from build123d import *

# Parameters (mm, degrees)
BOSS_EXTRUDE1_DEPTH = 6.25
SKETCH2_R           = 10
SKETCH2_R_2         = 5
BOSS_EXTRUDE2_DEPTH = 3
BOSS_EXTRUDE2_DRAFT = 10
SKETCH3_R           = 5
SKETCH3_R_2         = 10
CUT_EXTRUDE1_DEPTH  = 77.034531629
SKETCH5_R           = 40
BOSS_EXTRUDE3_DEPTH = 3.75
SKETCH6_R           = 15
CUT_EXTRUDE2_DEPTH  = 1
SKETCH7_R           = 17.5
CUT_EXTRUDE3_DEPTH  = 2
SKETCH8_R           = 15
CUT_EXTRUDE4_DEPTH  = 9
SKETCH11_R          = 4.5
CUT_EXTRUDE5_DEPTH  = 77.584920187
SKETCH13_R          = 8
CUT_EXTRUDE6_DEPTH  = 0.5
SKETCH14_R          = 2
CUT_EXTRUDE8_DEPTH  = 3
CHAMFER2_SIZE       = 0.5


with BuildPart() as part:
    # Sketch1 → Boss-Extrude1 (new, symmetric)
    with BuildSketch(Plane.XY):
        with BuildLine():
            Line((-36, -60), (36, -60))
            ThreePointArc((36, -60), (42.363961031, -57.363961031), (45, -51))
            Line((45, -51), (45, 51))
            ThreePointArc((45, 51), (42.363961031, 57.363961031), (36, 60))
            Line((36, 60), (-36, 60))
            ThreePointArc((-36, 60), (-42.363961031, 57.363961031), (-45, 51))
            Line((-45, 51), (-45, -51))
            ThreePointArc((-45, -51), (-42.363961031, -57.363961031), (-36, -60))
        make_face()
    extrude(amount=BOSS_EXTRUDE1_DEPTH, both=True)


with BuildPart() as boss_extrude2_tool:
    # Sketch2 → Boss-Extrude2 (with draft: the straight prism first)
    with BuildSketch(Plane(origin=(0, 0, -6.25), x_dir=(-1, 0, 0), z_dir=(0, 0, -1))):
        with BuildLine():
            ThreePointArc((42, 27.129319933), (41.019345657, 28.590440394), (39.987883834, 30.016148096))
            ThreePointArc((39.987883834, 30.016148096), (36.711412809, 37.344368202), (29.328259336, 40.495100991))
            ThreePointArc((29.328259336, 40.495100991), (0, 50), (-29.328259336, 40.495100991))
            ThreePointArc((-29.328259336, 40.495100991), (-36.711412809, 37.344368202), (-39.987883834, 30.016148096))
            ThreePointArc((-39.987883834, 30.016148096), (-41.019345657, 28.590440394), (-42, 27.129319933))
            Line((-42, 27.129319933), (-42, -27.129319933))
            ThreePointArc((-42, -27.129319933), (-41.019345657, -28.590440394), (-39.987883834, -30.016148096))
            ThreePointArc((-39.987883834, -30.016148096), (-36.711412809, -37.344368202), (-29.328259336, -40.495100991))
            ThreePointArc((-29.328259336, -40.495100991), (0, -50), (29.328259336, -40.495100991))
            ThreePointArc((29.328259336, -40.495100991), (36.711412809, -37.344368202), (39.987883834, -30.016148096))
            ThreePointArc((39.987883834, -30.016148096), (41.019345657, -28.590440394), (42, -27.129319933))
            Line((42, -27.129319933), (42, 27.129319933))
        make_face()
        with Locations((0, 15.2)):
            Circle(SKETCH2_R, mode=Mode.SUBTRACT)
        with Locations((29, 29.5)):
            Circle(SKETCH2_R_2, mode=Mode.SUBTRACT)
        with Locations((29, -29.5)):
            Circle(SKETCH2_R_2, mode=Mode.SUBTRACT)
        with Locations((-29, -29.5)):
            Circle(SKETCH2_R_2, mode=Mode.SUBTRACT)
        with Locations((-29, 29.5)):
            Circle(SKETCH2_R_2, mode=Mode.SUBTRACT)
    extrude(amount=BOSS_EXTRUDE2_DEPTH)
    # Boss-Extrude2: the draft: its side faces are tilted about the plane it starts from
    boss_extrude2_sides = [boss_extrude2_tool.faces().sort_by_distance(p)[0] for p in [
        (0, -50, -7.75),
        (-36.711412809, -37.344368202, -7.75),
        (-41.019345657, -28.590440394, -7.75),
        (-42, 0, -7.75),
        (-41.019345657, 28.590440394, -7.75),
        (-36.711412809, 37.344368202, -7.75),
        (0, 50, -7.75),
        (36.711412809, 37.344368202, -7.75),
        (41.019345657, 28.590440394, -7.75),
        (42, 0, -7.75),
        (41.019345657, -28.590440394, -7.75),
        (36.711412809, -37.344368202, -7.75),
        (10, 15.2, -7.75),
        (-24, 29.5, -7.75),
        (-24, -29.5, -7.75),
        (34, -29.5, -7.75),
        (34, 29.5, -7.75),
    ]]
    draft(boss_extrude2_sides, Plane(origin=(0, 0, -6.25), x_dir=(-1, 0, 0), z_dir=(0, 0, -1)), BOSS_EXTRUDE2_DRAFT)


with BuildPart() as part_1:
    add(part.part)

    # Boss-Extrude2: add boss_extrude2_tool
    add(boss_extrude2_tool.part)

    # Sketch3 → Cut-Extrude1 (cut, through all)
    with BuildSketch(Plane(origin=(0, 0, -6.25), x_dir=(-1, 0, 0), z_dir=(0, 0, -1))):
        with Locations((29, -29.5)):
            Circle(SKETCH3_R)
        with Locations((-29, -29.5)):
            Circle(SKETCH3_R)
        with Locations((29, 29.5)):
            Circle(SKETCH3_R)
        with Locations((-29, 29.5)):
            Circle(SKETCH3_R)
        with Locations((0, 15.2)):
            Circle(SKETCH3_R_2)
    extrude(amount=-CUT_EXTRUDE1_DEPTH, mode=Mode.SUBTRACT)

    # Sketch5 → Boss-Extrude3 (add, symmetric)
    with BuildSketch(Plane.XY.offset(6.25)):
        with Locations(Location((0, 15.2, 0), (0, 0, 180))):
            Circle(SKETCH5_R)
    extrude(amount=BOSS_EXTRUDE3_DEPTH, both=True)

    # Sketch6 → Cut-Extrude2 (cut)
    with BuildSketch(Plane.XY.offset(10)):
        with Locations((0, 15.2)):
            Circle(SKETCH6_R)
    extrude(amount=-CUT_EXTRUDE2_DEPTH, mode=Mode.SUBTRACT)

    # Sketch7 → Cut-Extrude3 (cut)
    with BuildSketch(Plane.XY.offset(9)):
        with Locations((0, 15.2)):
            Circle(SKETCH7_R)
    extrude(amount=-CUT_EXTRUDE3_DEPTH, mode=Mode.SUBTRACT)

    # Sketch8 → Cut-Extrude4 (cut)
    with BuildSketch(Plane.XY.offset(7)):
        with Locations((0, 15.2)):
            Circle(SKETCH8_R)
    extrude(amount=-CUT_EXTRUDE4_DEPTH, mode=Mode.SUBTRACT)

    # Sketch11 → Cut-Extrude5 (cut, through all)
    with BuildSketch(Plane.XY.offset(6.25)):
        with Locations((36, 51)):
            Circle(SKETCH11_R)
        with Locations(Location((-36, 51, 0), (0, 0, 180))):
            Circle(SKETCH11_R)
        with Locations(Location((36, -51, 0), (0, 0, 180))):
            Circle(SKETCH11_R)
        with Locations((-36, -51)):
            Circle(SKETCH11_R)
    extrude(amount=-CUT_EXTRUDE5_DEPTH, mode=Mode.SUBTRACT)

    # Sketch13 → Cut-Extrude6 (cut)
    with BuildSketch(Plane.XY.offset(6.25)):
        with Locations((36, 51)):
            Circle(SKETCH13_R)
        with Locations((-36, 51)):
            Circle(SKETCH13_R)
        with Locations((-36, -51)):
            Circle(SKETCH13_R)
        with Locations((36, -51)):
            Circle(SKETCH13_R)
    extrude(amount=-CUT_EXTRUDE6_DEPTH, mode=Mode.SUBTRACT)

    # Chamfer1: read off the stored shape, not the designer's step
    # Chamfer1 outline → Chamfer1 (revolve, cut)
    with BuildSketch(Plane.XZ.offset(-15.2)):
        Polygon((40, 10), (39.5, 10), (40, 9.5), align=None)
    revolve(axis=Axis((0, 15.2, 0), (0, 0, 1)), mode=Mode.SUBTRACT)

    # Sketch14 → Cut-Extrude8 (cut)
    with BuildSketch(Plane(origin=(0, 0, -9.25), x_dir=(-1, 0, 0), z_dir=(0, 0, -1))):
        with Locations((0, 39.5)):
            Circle(SKETCH14_R)
        with Locations(Location((0, -39.5, 0), (0, 0, 180))):
            Circle(SKETCH14_R)
    extrude(amount=-CUT_EXTRUDE8_DEPTH, mode=Mode.SUBTRACT)

    # Chamfer2
    chamfer2_edges = [part_1.edges().sort_by_distance(p)[0] for p in [
        (2, 39.5, -6.25),
        (-2, -39.5, -6.25),
    ]]
    chamfer(chamfer2_edges, length=CHAMFER2_SIZE)


solid = part_1.part
CAD build for the part. Positions are in the model's coordinates, mm. A direction names the side the tool comes from. Coordinates: 2 decimals unless noted, no trailing zeros. Answer as a JSON object with one key per item and string values. Group by question number.
1) Pin check, flat tips, straight feed: pin 1 Ø17.5 at (x, y) = (34.5, -53) entering from +Z; pin 2 Ø14.5 at (x, y) = (36, 51) entering from +Z; pin 3 Ø0.9 at (x, y) = (-0.5, -39) entering from -Z; pin 4 Ø4.5 at (x, y) = (0, -39.5) entering from -Z. Stop position of each tip, or through.
2) Tool access for faces 1 (the face through (13, 23, 9)), 2 (the face through (-37.041, 58.932, 6.004)), 3 (the face through (-29, 29, 2.5)): list every direction of +Z, -Z, +X, -X, +Y, -Y with a clear straight run to the whole face (end or side of a thin tool).
3) Saw through at A-A (z = -4.75). Give the number of separate pieces and of enclosed holes in the cut face, plus the area to 3 significant figures.
4) Mould opens along Z. For faces 4 (the face through (-36.406, -37.196, -8.062)), 5 (the face through (-32.6, -54.4, 5.75)), 6 (the face through (13, 23, 7)), 7 (the face through (-42.294, 57.434, 0.088)) say: +Z half, -Z half, draft (parallel to the pull), parting line (faces both ways), or undercut.
5) Wall check: line 1 (Y direction, x = -36, z = 6.1); line 2 (Y direction, x = -36, z = 0.5); line 3 (X direction, y = 48, z = 4.75). Give the ranges that are in metal, low to high. Write a range as from..to.
Values follow:
{
 "1": {"pin 1": "stops at z = 6.25", "pin 2": "stops at z = 5.75", "pin 3": "stops at z = -6.25", "pin 4": "stops at z = -9.25"},
 "2": {"face 1": "none", "face 2": "+Z", "face 3": "-Z"},
 "3": {"separate pieces": "1", "enclosed holes": "9", "area": "9,850 mm2"},
 "4": {"face 4": "-Z half", "face 5": "+Z half", "face 6": "undercut", "face 7": "draft"},
 "5": {"line 1": "y = -60..-59, -43..43, 59..60", "line 2": "y = -60..-55.5, -46.5..46.5, 55.5..60", "line 3": "x = -45..-39.35, -32.65..32.65, 39.35..45"}
}
